from build123d import *

# Parameters (mm, degrees)
SKETCH1_W                = 2400
SKETCH1_H                = 225
BOSS_EXTRUDE1_DEPTH      = 10
BOSS_EXTRUDE3_START      = 30
BOSS_EXTRUDE3_DEPTH      = 80
BOSS_EXTRUDE5_START      = 30
BOSS_EXTRUDE5_DEPTH      = 80
BOSS_EXTRUDE6_START      = -30
BOSS_EXTRUDE6_DEPTH      = 80
BOSS_EXTRUDE7_START      = 30
BOSS_EXTRUDE7_DEPTH      = 80
BOSS_EXTRUDE8_DEPTH      = 80
BOSS_EXTRUDE8_DEPTH_BACK = 140
BOSS_EXTRUDE8_START      = 30


with BuildPart() as part:
    # Sketch1 → Boss-Extrude1 (new body)
    with BuildSketch(Plane(origin=(0, 0, 0), x_dir=(1, 0, 0), z_dir=(0, 1, 0))):
        Rectangle(SKETCH1_W, SKETCH1_H)
    extrude(amount=BOSS_EXTRUDE1_DEPTH)

    # Sketch4 → Boss-Extrude3 (add)
    with BuildSketch(Plane.XY.offset(BOSS_EXTRUDE3_START)):
        Polygon((-1075, 10), (-900, 10), (-925, 40), (-1050, 40), align=None)
    extrude(amount=BOSS_EXTRUDE3_DEPTH)

    # Sketch6 → Boss-Extrude5 (add)
    with BuildSketch(Plane.XY.offset(BOSS_EXTRUDE5_START)):
        Polygon((-550, 40), (-575, 10), (-400, 10), (-425, 40), align=None)
    extrude(amount=BOSS_EXTRUDE5_DEPTH)

    # Sketch5 → Boss-Extrude6 (add)
    with BuildSketch(Plane.XY.offset(BOSS_EXTRUDE6_START)):
        Polygon((-75, 10), (100, 10), (75, 40), (-50, 40), align=None)
    extrude(amount=-BOSS_EXTRUDE6_DEPTH)

    # Sketch7 → Boss-Extrude7 (add)
    with BuildSketch(Plane.XY.offset(BOSS_EXTRUDE7_START)):
        Polygon((575, 40), (450, 40), (425, 10), (600, 10), align=None)
    extrude(amount=BOSS_EXTRUDE7_DEPTH)

    # Sketch8 → Boss-Extrude8 (add, two sides: drawn at the far end of the back side and taken through both)
    with BuildSketch(Plane.XY.offset(BOSS_EXTRUDE8_START - BOSS_EXTRUDE8_DEPTH_BACK)):
        Polygon((1075, 40), (950, 40), (925, 10), (1100, 10), align=None)
    extrude(amount=BOSS_EXTRUDE8_DEPTH + BOSS_EXTRUDE8_DEPTH_BACK)


solid = part.part
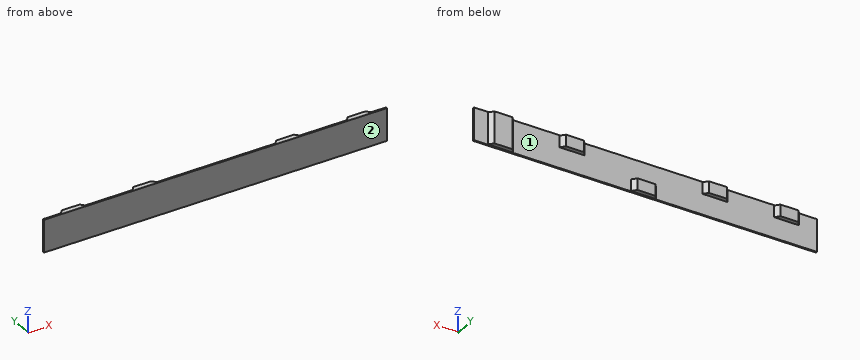
Can you work these out from the model? Positions are in its coordinate system, mm. Face numbers are marked on the shaded views. Coordinates: 2 decimals unless noted, no trailing zeros. Write each loop counter-clockwise with the first axis right and the second up, starting at its lowest first coordinate (ties: lowest second). Pieces come first, ordered by that corner, then holes. Notation, with made-up numbers: (44, 81) -> (48, 81) arc R27 ccw to (48, 106) -> close; hole circle Ø4 at (41, 8.25). An arc over 180 degrees is marked (long way). Write each question's results on one line, items separated by ' | '. Start each with the question number.
Q1. Imagine slicing it at D-D (x = -973). Write out the boundary of the cut face in (y, z).
Q2. Imagine slicing it at A-A (y = 16). Write out the boundary of the cut face in (x, z), then the cut area to 3 significant figures.
Q3. We'd pull the mould along X, two halves only. Please class the marked faces 1 and 2: +X half, -X half, draft (parallel to the pull), parting line (faces both ways), or undercut.
Q4. Imagine slicing it at B-B (z = 52). Write out the boundary of the cut face in (x, y).
Q5. Imagine slicing it at C-C (x = 992). Write out the boundary of the cut face in (y, z).
Q6. If I drill on probe 1 along X at (y, z) = (14.5, 74.5); probe 2 along X at (y, z) = (35.5, 33); probe 3 along Y at (x, z) = (423.5, -51), over which ranges is the centre line in solid material (lowest first)?
Q7. I'm going to push flat-ended pins straight in: pin 1 (15 mm diameter, centred on x = 1019.5, y = 28, fed in from +Z); pin 2 (2 mm diameter, centred on x = 214, z = -50, fed in from +Y); pin 3 (4 mm diameter, centred on y = 17, z = 78.5, fed in from -X); pin 4 (5 mm diameter, centred on x = -119, z = 89.5, fed in from -Y). Where does each tip first touch, or does it pass through?
Taken from the geometry:
1) outline: (0, -112.5) -> (10, -112.5) -> (10, 30) -> (40, 30) -> (40, 110) -> (10, 110) -> (10, 112.5) -> (0, 112.5) -> close
2) outline: (-1070, 30) -> (-905, 30) -> (-905, 110) -> (-1070, 110) -> close; (-570, 30) -> (-405, 30) -> (-405, 110) -> (-570, 110) -> close; (-70, -110) -> (95, -110) -> (95, -30) -> (-70, -30) -> close; (430, 30) -> (595, 30) -> (595, 110) -> (430, 110) -> close; (930, -110) -> (1095, -110) -> (1095, 110) -> (930, 110) -> close | area: 89,100 mm^2
3) face 1: undercut | face 2: draft
4) outline: (-1200, 0) -> (1200, 0) -> (1200, 10) -> (1100, 10) -> (1075, 40) -> (950, 40) -> (925, 10) -> (600, 10) -> (575, 40) -> (450, 40) -> (425, 10) -> (-400, 10) -> (-425, 40) -> (-550, 40) -> (-575, 10) -> (-900, 10) -> (-925, 40) -> (-1050, 40) -> (-1075, 10) -> (-1200, 10) -> close
5) outline: (0, -112.5) -> (10, -112.5) -> (10, -110) -> (40, -110) -> (40, 110) -> (10, 110) -> (10, 112.5) -> (0, 112.5) -> close
6) probe 1: x = -1071.25 to -903.75, -571.25 to -403.75, 428.75 to 596.25, 928.75 to 1096.25 | probe 2: x = -1053.75 to -921.25, -553.75 to -421.25, 446.25 to 578.75, 946.25 to 1078.75 | probe 3: y = 0 to 10
7) pin 1: stops at z = 110 | pin 2: stops at y = 10 | pin 3: stops at x = -1070.83 | pin 4: stops at y = 0
